Source: three-view drawing plus pictorial views. Frame: mm from the lowest corner of the part. A direction names the side the tool comes from. Coordinates: 2 decimals unless noted, no trailing zeros. Write each loop counter-clockwise with the first axis right and the second up, starting at its lowest first coordinate (ties: lowest second). Pieces come first, ordered by that corner, then holes. Notation, with made-up numbers: M 59,77 L 115,77 A17 ccw 115,104 Z; hole C -13.5,70 d10. An arc over 180 degrees is marked long. Answer as a JSON object with one key per item and string values. Group by question number.
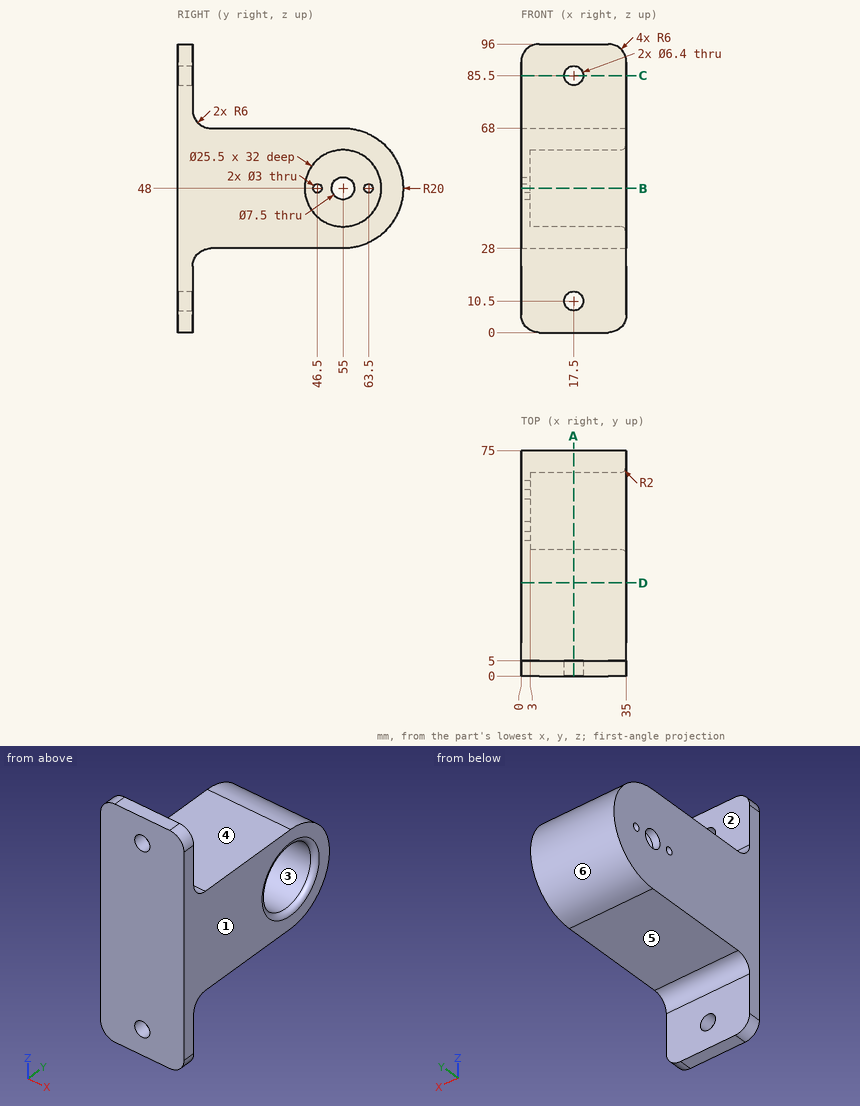
Q1. Section A-A, the plane x = 17.5. Return the cut outline in (y, z).
Q2. Section C-C, the plane z = 85.5. Return the cut outline in (x, y).
Q3. Pin query (flat end, axial travel): pin 1 Ø1 at (x, y) = (3.5, 48) entering from -Z; pin 2 Ø5 at (x, z) = (24.5, 59) entering from -Y; pin 3 Ø6.5 at (x, z) = (22.5, 80.5) entering from +Y; pin 4 Ø1 at (x, y) = (30, 65) entering from -Z. Return the tip coordinate at first contact, or that it passes through.
Q4. Section B-B, the plane z = 48. Return the cut outline in (x, y), and give its area (3 significant figures).
Q5. Line query: line 1 (Y direction, x = 2, z = 48); line 2 (Y direction, x = 21, z = 48); line 3 (Y direction, x = 21, z = 14). Output: solid intervals per line, ascending. Write a range as from..to.
Q6. Section D-D, the plane y = 31. Return the cut outline in (x, z), and give its area (3 significant figures).
Q7. Draft query along Y for the marked faces 1, 2 and 3. Return one class per face: released by +Y, released by -Y, zero draft, split by the parting line, or undercut.
Q8. Access query for the marked faces 4, 5 and 6. Directions: +Z, -Z, +X, -X, +Y, -Y. A direction counts if a zero-diameter tool reaches every point of the face in a straight line with its end or side. Return the directions, or none.
Filled in:
{
 "1": {"outline": "M 0,0 L 5,0 L 5,7.3 L 0,7.3 Z; M 0,13.7 L 5,13.7 L 5,22 A6 cw 11,28 L 55,28 A20 ccw 55,68 L 11,68 A6 cw 5,74 L 5,82.3 L 0,82.3 Z; M 0,88.7 L 5,88.7 L 5,96 L 0,96 Z; hole C 55,48 d25.5"},
 "2": {"outline": "M 0,0 L 14.3,0 L 14.3,5 L 0,5 Z; M 20.7,0 L 35,0 L 35,5 L 20.7,5 Z"},
 "3": {"pin 1": "z = 28", "pin 2": "y = 0", "pin 3": "y = 5", "pin 4": "z = 30.4"},
 "4": {"outline": "M 0,0 L 35,0 L 35,40.25 A2 ccw 33,42.25 L 3,42.25 L 3,45 L 0,45 Z; M 0,48 L 3,48 L 3,51.25 L 0,51.25 Z; M 0,58.75 L 3,58.75 L 3,62 L 0,62 Z; M 0,65 L 3,65 L 3,67.75 L 33,67.75 A2 ccw 35,69.75 L 35,75 L 0,75 Z", "area": "1,770 mm^2"},
 "5": {"line 1": "0..45, 48..51.25, 58.75..62, 65..75", "line 2": "0..42.25, 67.75..75", "line 3": "0..5"},
 "6": {"outline": "M 0,28 L 35,28 L 35,68 L 0,68 Z", "area": "1,400 mm^2"},
 "7": {"face 1": "zero draft", "face 2": "released by +Y", "face 3": "undercut"},
 "8": {"face 4": "+Z, +X, -X, +Y", "face 5": "-Z, +X, -X, +Y", "face 6": "+X, -X, +Y"}
}
